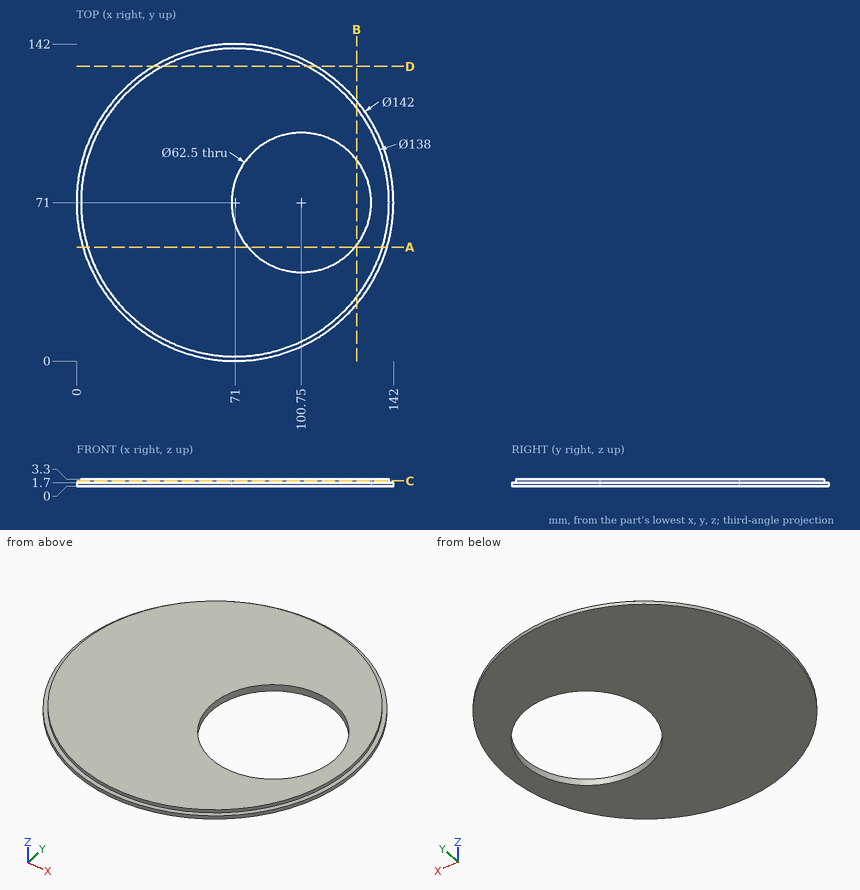
Check sheet for the drawn part. Datum: minimum x, y, z corner. Units: mm. Round coordinates to 2 decimals unless told otherwise and drop trailing zeros. Loops run counter-clockwise (first coordinate to the right, second up) from the corner with the lowest first, then second, coordinate; pieces in that order, holes last.
Item 1: Cross-section at D-D on y = 132. Record the boundary of the cut face in (x, z), then the cut area to 3 significant figures.
Item 2: Cross-section at B-B on x = 125.5. Record the boundary of the cut face in (y, z), then the cut area to 3 significant figures.
Item 3: Cross-section at A-A on y = 51. Record the boundary of the cut face in (x, z), then the cut area to 3 significant figures.
Item 4: Cross-section at C-C on z = 2.45. Record the boundary of the cut face in (x, y).
Item 5: Thickness scan on line 1 (Y direction, x = 81, z = 0.65); line 2 (X direction, y = 96.5, z = 2.1); line 3 (X direction, y = 79, z = 2.4). Record the ranges inside material, lowest first.
Item 6: Gauge pin test, flat end, axial feed: pin 1 (1.5 mm diameter, centred on x = 49, z = 2, fed in from +Y). Record the tip position at first contact, or that the pin passes through.
Answer sheet:
1. outline: (34.67, 0) - (107.33, 0) - (107.33, 1.7) - (103.25, 1.7) - (103.25, 3.3) - (38.75, 3.3) - (38.75, 1.7) - (34.67, 1.7) - close
1. area: 227 mm2
2. outline: (25.49, 0) - (51.92, 0) - (51.92, 3.3) - (28.68, 3.3) - (28.68, 1.7) - (25.49, 1.7) - close; (90.08, 0) - (116.51, 0) - (116.51, 1.7) - (113.32, 1.7) - (113.32, 3.3) - (90.08, 3.3) - close
2. area: 164 mm2
3. outline: (2.88, 0) - (76.74, 0) - (76.74, 3.3) - (4.96, 3.3) - (4.96, 1.7) - (2.88, 1.7) - close; (124.76, 0) - (139.12, 0) - (139.12, 1.7) - (137.04, 1.7) - (137.04, 3.3) - (124.76, 3.3) - close
3. area: 284 mm2
4. outline: circle Ø138 at (71, 71); hole circle Ø62.5 at (100.75, 71)
5. line 1: y = 0.71 to 46.78, 95.22 to 141.29
5. line 2: x = 6.88 to 82.69, 118.81 to 135.12
5. line 3: x = 2.47 to 70.54, 130.96 to 139.53
6. pin 1: stops at y = 138.73
